Verification items for the finished model (mm, model axes). Face numbers are marked on the shaded views. Give positions to 0.01 mm unless a question says otherwise; leave off trailing zeros. Loops run counter-clockwise (first coordinate to the right, second up) from the corner with the lowest first, then second, coordinate; pieces in that order, holes last. Notation, with made-up numbers: M -12.5,33.25 L 5.5,33.25 A26 cw 5.5,70.25 Z; hole C -2,7.5 d6. An arc over 180 degrees is marked long. Use a Markdown table: item, result.
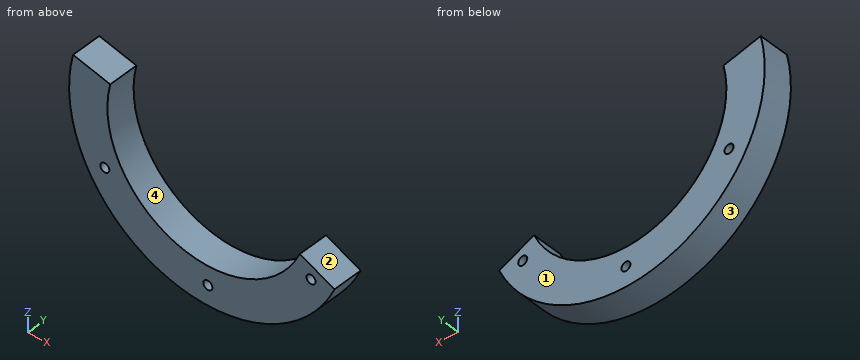
from build123d import *

# Parameters (mm, degrees)
SKETCH1_R           = 46.0375
SKETCH1_R_2         = 1.5
SKETCH1_R_3         = 33.3375
BOSS_EXTRUDE1_DEPTH = 10
CUT_EXTRUDE1_DEPTH  = 66.870348508


with BuildPart() as part:
    # Sketch1 → Boss-Extrude1 (new body)
    with BuildSketch(Plane(origin=(0, 0, 0), x_dir=(1, 0, 0), z_dir=(0, 1, 0))):
        with Locations(Location((0, 0, 0), (0, 0, 270))):
            Circle(SKETCH1_R)
        with Locations(Location((0, 39.5, 0), (0, 0, 270))):
            Circle(SKETCH1_R_2, mode=Mode.SUBTRACT)
        with Locations(Location((34.208003449, 19.75, 0), (0, 0, 270))):
            Circle(SKETCH1_R_2, mode=Mode.SUBTRACT)
        with Locations(Location((34.208003449, -19.75, 0), (0, 0, 270))):
            Circle(SKETCH1_R_2, mode=Mode.SUBTRACT)
        with Locations(Location((0, -39.5, 0), (0, 0, 270))):
            Circle(SKETCH1_R_2, mode=Mode.SUBTRACT)
        with Locations(Location((-34.208003449, -19.75, 0), (0, 0, 270))):
            Circle(SKETCH1_R_2, mode=Mode.SUBTRACT)
        with Locations(Location((-34.208003449, 19.75, 0), (0, 0, 270))):
            Circle(SKETCH1_R_2, mode=Mode.SUBTRACT)
        with Locations(Location((0, 0, 0), (0, 0, 270))):
            Circle(SKETCH1_R_3, mode=Mode.SUBTRACT)
    extrude(amount=BOSS_EXTRUDE1_DEPTH)

    # Sketch2 → Cut-Extrude1 (cut, through all)
    with BuildSketch(Plane(origin=(0, 10, 0), x_dir=(1, 0, 0), z_dir=(0, 1, 0))):
        with BuildLine():
            Line((0, 0), (-44.72616408, -10.909704529))
            ThreePointArc((-44.72616408, -10.909704529), (14.909439021, -43.556400613), (42.029747553, 18.787009525))
            Line((42.029747553, 18.787009525), (0, 0))
        make_face()
    extrude(amount=-CUT_EXTRUDE1_DEPTH, mode=Mode.SUBTRACT)


solid = part.part
(1) Cross-section at B-B on z = -25.5. Record the cut outline in (x, y), then the cut area to 3 significant figures.
Results below:
| item | result |
|---|---|
| outline | M -38.33,0 L -21.47,0 L -21.47,10 L -38.33,10 Z; M 21.47,0 L 38.33,0 L 38.33,10 L 21.47,10 Z |
| area | 337 mm^2 |
(2) Material ranges on line 1 (X direction, y = 6, z = -20); line 2 (X direction, y = 3.75, z = -19.75); line 3 (X direction, y = 4, z = -39), recorded low to high.
Results below:
| item | result |
|---|---|
| line 1 | -41.47 to -35.69, -32.73 to -26.67, 26.67 to 32.73, 35.69 to 41.47 |
| line 2 | -41.59 to -35.71, -32.71 to -26.86, 26.86 to 32.71, 35.71 to 41.59 |
| line 3 | -24.46 to -1.41, 1.41 to 24.46 |
(3) Cross-section at A-A on x = 0. Record the cut outline in (y, z), then the cut area to 3 significant figures.
Results below:
| item | result |
|---|---|
| outline | M 0,-46.04 L 10,-46.04 L 10,-41 L 0,-41 Z; M 0,-38 L 10,-38 L 10,-33.34 L 0,-33.34 Z |
| area | 97.0 mm^2 |
(4) Gauge pin test, flat ends, axial feed: P1, Ø1, axis at y = 3.5, z = 2.5, coming from the +X side; P2, Ø6, axis at y = 9, z = 5, coming from the -X side; P3, Ø6, axis at y = 2.5, z = 4.5, coming from the +X side. Record the tip position at first contact, or that the pin passes through.
Results below:
| item | result |
|---|---|
| P1 | x = -33.2 |
| P2 | x = -45.99 |
| P3 | x = -32.48 |
(5) Cross-section at C-C on z = -19.75. Record the cut outline in (x, y), then the cut area to 3 significant figures.
Results below:
| item | result |
|---|---|
| outline | M -41.59,0 L -35.71,0 L -35.71,10 L -41.59,10 Z; M -32.71,0 L -26.86,0 L -26.86,10 L -32.71,10 Z; M 26.86,0 L 32.71,0 L 32.71,10 L 26.86,10 Z; M 35.71,0 L 41.59,0 L 41.59,10 L 35.71,10 Z |
| area | 235 mm^2 |
(6) Cross-section at D-D on y = 2.75. State how many separate pieces and enclosed holes the cut face has, then the cut area to 3 significant figures.
Results below:
| item | result |
|---|---|
| separate pieces | 1 |
| enclosed holes | 3 |
| area | 1,470 mm^2 |
(7) Draft check along X on the marked faces 1, 2, 3 and 4. Enter one of: +X half, -X half, draft (parallel to the pull), parting line (faces both ways), or undercut.
Results below:
| item | result |
|---|---|
| face 1 | draft |
| face 2 | +X half |
| face 3 | parting line |
| face 4 | undercut |
